Check sheet for the modelled part. Datum: model origin and axes. Units: mm. A direction names the side the tool comes from. Give positions to 0.01 mm unless a question says otherwise; leave off trailing zeros. Order: outer loops, then holes, each group sorted by start corner. A loop starts at its lowest first (then second) coordinate and runs counter-clockwise, first axis right, second up. Notation, with made-up numbers: M -24.5,12 L -7.5,12 A26 ccw -7.5,29 Z; hole C -27,8.25 d5. An arc over 180 degrees is marked long. Answer in a Markdown table with one row per item. Add a question column.
from build123d import *

# Parameters (mm, degrees)
F0_R      = 5.75
F0_R_2    = 4
F1_DEPTH  = 3
F3_R      = 3.5
F4_DEPTH  = 17
F5_W      = 20
F5_H      = 5.5
F6_DEPTH  = 25
F12_DEPTH = 6
F10_R     = 2.5
F13_DEPTH = 25


with BuildPart() as f1:
    # F0 (on Front) → F1 (new body, symmetric)
    with BuildSketch(Plane.XZ):
        Circle(F0_R)
        Circle(F0_R_2, mode=Mode.SUBTRACT)
    extrude(amount=F1_DEPTH, both=True)

    # F3 (on offset) → F4 (join)
    with BuildSketch(Plane.YZ.offset(4.5)):
        Circle(F3_R)
    extrude(amount=F4_DEPTH)

    # F5 (on face) → F6 (cut)
    with BuildSketch(Plane.XZ.offset(3)):
        with Locations((-10, 0)):
            Rectangle(F5_W, F5_H)
    extrude(amount=-F6_DEPTH, mode=Mode.SUBTRACT)

    # F11 (on face) → F12 (join)
    with BuildSketch(Plane.XZ.offset(3)):
        Polygon((15, 2), (0, 5.75), (4.887585, 1.127019), (4.887585, -0.959626), (0, -5.75), (15, -2), align=None)
    extrude(amount=-F12_DEPTH)

    # F10 (on face) → F13 (cut)
    with BuildSketch(Plane.YZ.offset(21.5)):
        Circle(F10_R)
    extrude(amount=-F13_DEPTH, mode=Mode.SUBTRACT)


solid = f1.part
Q1. Thickness scan on probe 1 along Z at (x, y) = (16, 0); probe 2 along Z at (x, y) = (0, 0). Record the ranges inside material, lowest first.
Q2. Tool access check on faces 5 (the cylindrical face through (14.77, 3.233, -1.341)), 6 (the cylindrical face through (1.84, 0.04, -3.55)), 7 (the flat face through (-4, 0, -2.75)). Record the directions out of +Z, -Z, +X, -X, +Y, -Y that give a thin tool (end or side, any length) a straight path to the whole face; none if there is none.
Q3. Go/stop test with flat-tipped pins: pin 1 (0.6 mm diameter, centred on y = -3, z = 0, fed in from -X); pin 2 (1.7 mm diameter, centred on x = -4, y = 0, fed in from -Z); pin 3 (2 mm diameter, centred on x = -2, y = -1, fed in from -Z). Record where each tip stops, or that it passes through.
Q4. Cross-section at D-D (x = 11). Record the boundary of the cut face in (y, z).
Q5. Cross-section at A-A (y = 0). Record the boundary of the cut face in (x, z), and give its area (3 significant figures).
Q6. Cross-section at C-C (z = -0.5). Record the boundary of the cut face in (x, y), and give its area (3 significant figures).
Q7. Draft check along Z on faces 1 (the flat face through (-4, 0, 2.75)), 2 (the cylindrical face through (-1.59, -0.042, 5.526)), 3 (the cylindrical face through (12.44, -0.54, -2.44)), 4 (the cylindrical face through (-1.71, -0.04, -5.49)). Enter one of: pulls with the +Z half, pulls with the -Z half, needs draft (parallel to the pull), parting line crosses it, or undercut.
Q8. Cross-section at B-B (x = 0). Record the boundary of the cut face in (y, z).
Values follow:
| question | item | result |
|---|---|---|
| 1 | probe 1 | -3.5 to -2.5, 2.5 to 3.5 |
| 1 | probe 2 | -5.75 to -4, 4 to 5.75 |
| 2 | face 5 | +X |
| 2 | face 6 | +Y, -Y |
| 2 | face 7 | -X, +Y, -Y |
| 3 | pin 1 | x = 3.99 |
| 3 | pin 2 | z = -4.81 |
| 3 | pin 3 | z = -5.66 |
| 4 | outline | M -3,-3 L -1.8,-3 A3.5 ccw 1.8,-3 L 3,-3 L 3,-1.8 A3.5 ccw 3,1.8 L 3,3 L 1.8,3 A3.5 ccw -1.8,3 L -3,3 L -3,1.8 A3.5 ccw -3,-1.8 Z; hole C 0,0 d5 |
| 5 | outline | M -5.05,-2.75 A5.75 ccw 2.71,-5.07 L 9,-3.5 L 21.5,-3.5 L 21.5,-2.5 L 3.12,-2.5 A4 cw -2.9,-2.75 Z; M -5.05,2.75 L -2.9,2.75 A4 cw 3.12,2.5 L 21.5,2.5 L 21.5,3.5 L 9,3.5 L 2.71,5.07 A5.75 ccw Z |
| 5 | area | 73.9 mm² |
| 6 | outline | M 3.97,-3 L 4.5,-3 L 4.5,-3.46 L 21.5,-3.46 L 21.5,-2.45 L 3.97,-2.45 Z; M 3.97,2.45 L 21.5,2.45 L 21.5,3.46 L 4.5,3.46 L 4.5,3 L 3.97,3 Z |
| 6 | area | 35.1 mm² |
| 7 | face 1 | undercut |
| 7 | face 2 | pulls with the +Z half |
| 7 | face 3 | undercut |
| 7 | face 4 | pulls with the -Z half |
| 8 | outline | M -3,-5.75 L 3,-5.75 L 3,-4 L -3,-4 Z; M -3,4 L 3,4 L 3,5.75 L -3,5.75 Z |
